Design review of the part built by this model. Coordinates are the model's own, in mm. Face numbers are marked on the shaded views. A direction names the side the tool comes from. Coordinates: 2 decimals unless noted, no trailing zeros. Loops run counter-clockwise (first coordinate to the right, second up) from the corner with the lowest first, then second, coordinate; pieces in that order, holes last. Notation, with made-up numbers: M 82,-38 L 133,-38 A21 ccw 133,0 Z; hole C 29.5,48.5 d3. An arc over 180 degrees is marked long. Write item = value, one per line. Start each with the question number.
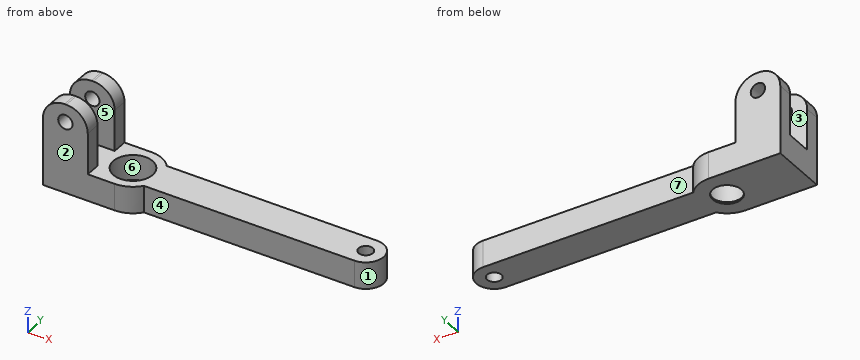
Autodesk Inventor part; units mm, degrees
ref_plane "YZ Plane" through (0, 0, 0) normal (1, 0, 0) x (0, 1, 0)
ref_plane "XZ Plane" through (0, 0, 0) normal (0, 1, 0) x (-1, 0, 0)
ref_plane "XY Plane" through (0, 0, 0) normal (0, 0, 1) x (1, 0, 0)
sketch "Sketch1" plane through (0, 0, 0) normal (0, 0, 1) x (1, 0, 0)
  line L0 (0, 0) -> (-40, 0) construction
  line L1 (0, 16) -> (-40, 16)
  line L2 (-40, -16) -> (0, -16)
  arc A0 (0, -16) -> (0, 16) centre (0, 0) ccw
  arc A1 (-40, 16) -> (-40, -16) centre (-40, 0) ccw construction
  circle A2 centre (0, 0) radius 11
  line L3 (-40, 16) -> (-40, -16)
  point P0 (-20, 0)
  dimension "d0" = 22
  dimension "d1" = 5
  dimension "d2" = 40
extrude "Extrusion1" add sketch "Sketch1" along normal blind 15
sketch "Sketch2" plane through (0, 0, 15) normal (0, 0, 1) x (1, 0, 0)
  line L0 (0, 16) -> (-40, 16)
  line L1 (-40, 16) -> (-15, 16)
  line L2 (-15, 16) -> (-15, 7.5)
  line L3 (-15, 7.5) -> (-40, 7.5)
  line L4 (-40, 7.5) -> (-40, 16)
  line L5 (-40, 16) -> (-40, -16)
  line L6 (-40, -16) -> (-15, -16)
  line L7 (-15, -16) -> (-15, -7.5)
  line L8 (-15, -7.5) -> (-40, -7.5)
  line L9 (-40, -7.5) -> (-40, -16)
  point P0 (0, 0)
  dimension "d5" = 25
  dimension "d6" = 15
extrude "Extrusion2" add sketch "Sketch2" along normal blind 35
sketch "Sketch3" plane through (-40, -16, 0) normal (0, -1, 0) x (1, 0, 0)
  line L0 (0, 15) -> (25, 15)
  line L1 (0, 50) -> (25, 50) construction
  line L2 (12.5, 50) -> (12.5, 40) construction
  circle A0 centre (12.5, 40) radius 4
  point P0 (40, 0)
  dimension "d9" = 8
  dimension "d10" = 10
extrude "Extrusion3" cut sketch "Sketch3" against normal through all
fillet "Fillet1" radius 12 4 edges at (-15, 11.75, 50) (-40, 11.75, 50) (-15, -11.75, 50) (-40, -11.75, 50)
sketch "Sketch4" plane through (0, 0, 0) normal (0, 0, -1) x (-1, 0, 0)
  circle A0 centre (0, 0) radius 11
  circle A1 centre (0, 0) radius 8
  dimension "d14" = 16
extrude "Extrusion4" add sketch "Sketch4" against normal blind 1
sketch "Sketch5" plane through (0, 0, 0) normal (0, 0, -1) x (-1, 0, 0)
  arc A0 (-120, 50) -> (-120, -50) centre (0, 0) ccw construction
  line L0 (0, 0) -> (-120, 50) construction
  circle A1 centre (0, 0) radius 11 construction
  line L1 (0, 0) -> (-120, -50) construction
  line L2 (0, 0) -> (-130, 0) construction
  line L3 (-120, 50) -> (-120, -50) construction
  line L4 (0, 0) -> (-130, 0) construction
  line L5 (0, 10) -> (-12.49, 10)
  line L6 (-130, -10) -> (-12.49, -10)
  arc A2 (0, -10) -> (0, 10) centre (0, 0) ccw
  arc A3 (-130, 10) -> (-130, -10) centre (-130, 0) ccw
  circle A4 centre (-130, 0) radius 4
  arc A5 (0, 16) -> (0, -16) centre (0, 0) ccw
  arc A6 (-12.49, 10) -> (-12.49, -10) centre (0, 0) ccw
  line L7 (-12.49, 10) -> (-130, 10)
  line L8 (-12.49, -10) -> (0, -10)
  point P0 (-65, 0)
  dimension "d17" = 100
  dimension "d18" = 130
  dimension "d19" = 45.24
  dimension "d20" = 10
  dimension "d21" = 8
extrude "Extrusion5" add sketch "Sketch5" against normal up to surface (15 mm away) contours A5 L6 A3 L7
properties part number "tiller rotation bracket"
Q1. Add section D-D on y = -14. State the section outline as (x, z) points, plus the area to 3 significant figures.
Q2. Add section B-B on y = 0. State the section outline as (x, z) points.
Q3. Clearance check with flat-ended pins moving along their axes: P1, Ø1.5, axis at y = -12, z = 25.5, coming from the +X side; P2, Ø3, axis at y = -4.5, z = 24.5, coming from the -X side; P3, Ø1.5, axis at x = -18.5, y = 11.5, coming from the +Z side; P4, Ø17.5, axis at x = 0.5, y = -3.5, coming from the +Z side. State where each tip first meets the part, or that it passes through.
Q4. Add section A-A on z = 28. State the section outline as (x, y) points.
Q5. To check wall thickness, follow line 1 (Y direction, x = 0, z = 9); line 2 (Y direction, x = 130, z = 7.5); line 3 (Z direction, x = 89, y = -9.5). State the ranges of each line that lie inside material, in increasing order. Write a range as from..to.
Q6. For the marked faces 4, 5, 6 and 7, list the 3-axis set-ups (+Z, -Z, +X, -X, +Y, -Y) from which the entire face can be reached by the end or side of a thin tool; tool diameter is ignored.
Q7. Add section C-C on z = 7. State the section outline as (x, y) points, plus the area to 3 significant figures.
Q8. Mouldability with a two-part tool opening along Y and no side actions: class the marked faces 1, 2 and 3 as released by +Y, released by -Y, zero draft, split by the parting line, or undercut.
Values follow:
q1.outline = M -40,0 L 7.75,0 L 7.75,15 L -15,15 L -15,38 A12 ccw -27,50 L -28,50 A12 ccw -40,38 Z; hole C -27.5,40 d8
q1.area = 1,480 mm2
q2.outline = M -40,0 L -8,0 L -8,1 L -11,1 L -11,15 L -40,15 Z; M 8,0 L 126,0 L 126,15 L 11,15 L 11,1 L 8,1 Z; M 134,0 L 140,0 L 140,15 L 134,15 Z
q3.P1 = -15
q3.P2 = through
q3.P3 = 47.16
q3.P4 = 15
q4.outline = M -40,-16 L -15,-16 L -15,-7.5 L -40,-7.5 Z; M -40,7.5 L -15,7.5 L -15,16 L -40,16 Z
q5.line_1 = -16..-11, 11..16
q5.line_2 = -10..-4, 4..10
q5.line_3 = 0..15
q6.face_4 = +Z, -Z, +X, -Y
q6.face_5 = +Z, +X, -X
q6.face_6 = +Z
q6.face_7 = +Z, -Z, +X, +Y
q7.outline = M -40,-16 L 0,-16 A16 ccw 12.49,-10 L 130,-10 A10 ccw 130,10 L 12.49,10 A16 ccw 0,16 L -40,16 Z; hole C 0,0 d22; hole C 130,0 d8
q7.area = 3,710 mm2
q8.face_1 = split by the parting line
q8.face_2 = released by -Y
q8.face_3 = undercut
